Source: CAD feature listing. Evaluate the final solid. Frame: model axes, mm. A direction names the side the tool comes from. Give positions to 0.01 mm unless a question says otherwise; leave off trailing zeros. Write each loop counter-clockwise with the first axis right and the second up, starting at its lowest first coordinate (ties: lowest second). Pieces come first, ordered by that corner, then holes. Notation, with made-up numbers: (83.25, 41.5) -> (108.25, 41.5) arc R21 ccw to (108.25, 61.5) -> close; hole circle Ø8 at (-22.75, 50.25). An arc over 180 degrees is marked (long way). Answer as a JSON object with one key per item and string values. Group by question number.
Item 1: Pull-direction query (X, two-part tool) for faces 1 (the face through (25, 4, -7)), 2 (the face through (0, 7, 7)), 3 (the face through (14, 0, -5)); classes: pulls with the +X half, pulls with the -X half, needs draft (parallel to the pull), parting line crosses it, or undercut.
Item 2: Section query C-C on y = 7. Return the cut outline in (x, z).
Item 3: Access query for faces 4 (the face through (22, 12, -4)), 5 (the face through (40, 7, -6)), 6 (the face through (2.465, 5.388, 17.547)), 7 (the face through (25, 9.5, -8)), 8 (the face through (12.5, 7, -5)). Directions: +Z, -Z, +X, -X, +Y, -Y. A direction counts if a zero-diameter tool reaches every point of the face in a straight line with its end or side. Return the directions, or none.
Item 4: Section query A-A on x = 27. Return the cut outline in (y, z).
Item 5: Ray query, probe 1 along Y at (x, z) = (1.4, 3.65); probe 2 along X at (y, z) = (11, -3); probe 3 along Z at (x, y) = (31.5, 3). Return the intervals inside material, ascending. Write a range as from..to.
Item 6: First-contact query: pin 1 Ø1.6 at (x, z) = (29, -7.5) entering from -Y; pin 2 Ø5 at (y, z) = (7, 3.65) entering from +X; pin 3 Ø1.5 at (x, y) = (15.5, 4) entering from +Z; pin 4 Ø4 at (y, z) = (4, 12.5) entering from +X. Flat tips, straight axial feed; report the tip coordinate or a pass-through.
Item 7: Section query D-D on z = -5.5. Return the cut outline in (x, y), plus the area to 3 significant figures.
Item 8: Section query B-B on z = 3.65. Return the cut outline in (x, y).
from build123d import *

# Parameters (mm, degrees)
BOSS_EXTRUDE1_DEPTH  = 14
SKETCH2_W            = 25
SKETCH2_H            = 7
CUT_EXTRUDE3_DEPTH   = 3
SKETCH10_W           = 18
SKETCH10_H           = 5
CUT_EXTRUDE4_DEPTH   = 43.95346319
SKETCH20_W           = 24
SKETCH20_H           = 14
BOSS_EXTRUDE10_DEPTH = 5
SKETCH21_R           = 2.65
CUT_EXTRUDE13_DEPTH  = 5
SKETCH22_W           = 5
SKETCH22_H           = 4
CUT_EXTRUDE14_DEPTH  = 49.703182648
SKETCH23_R           = 2.65
BOSS_EXTRUDE11_DEPTH = 5


with BuildPart() as part:
    # Sketch1 → Boss-Extrude1 (new body)
    with BuildSketch(Plane(origin=(0, 0, 0), x_dir=(1, 0, 0), z_dir=(0, 1, 0))):
        Polygon((6.589095597, 0), (10, 0), (10, 4), (40, 4), (40, 9), (11.589095597, 9), (0, 9), (0, 0), align=None)
    extrude(amount=BOSS_EXTRUDE1_DEPTH)

    # Sketch2 → Cut-Extrude3 (cut)
    with BuildSketch(Plane.XY.offset(-4)):
        with Locations((25, 7)):
            Rectangle(SKETCH2_W, SKETCH2_H)
    extrude(amount=-CUT_EXTRUDE3_DEPTH, mode=Mode.SUBTRACT)

    # Sketch10 → Cut-Extrude4 (cut, through all)
    with BuildSketch(Plane.XY.offset(-7)):
        with Locations((25, 7)):
            Rectangle(SKETCH10_W, SKETCH10_H)
    extrude(amount=-CUT_EXTRUDE4_DEPTH, mode=Mode.SUBTRACT)

    # Sketch20 → Boss-Extrude10 (add)
    with BuildSketch(Plane.ZY):
        with Locations((12, 7)):
            Rectangle(SKETCH20_W, SKETCH20_H)
    extrude(amount=-BOSS_EXTRUDE10_DEPTH)

    # Sketch21 → Cut-Extrude13 (cut)
    with BuildSketch(Plane.ZY):
        with Locations((-4.35, 7)):
            Circle(SKETCH21_R)
        with Locations((3.65, 7)):
            Circle(SKETCH21_R)
        with Locations((11.65, 7)):
            Circle(SKETCH21_R)
        with Locations((19.65, 7)):
            Circle(SKETCH21_R)
    extrude(amount=-CUT_EXTRUDE13_DEPTH, mode=Mode.SUBTRACT)

    # Sketch22 → Cut-Extrude14 (cut, through all)
    with BuildSketch(Plane(origin=(0, 14, 0), x_dir=(1, 0, 0), z_dir=(0, 1, 0))):
        with Locations((7.5, 2)):
            Rectangle(SKETCH22_W, SKETCH22_H)
    extrude(amount=-CUT_EXTRUDE14_DEPTH, mode=Mode.SUBTRACT)

    # Sketch23 → Boss-Extrude11 (add)
    with BuildSketch(Plane.ZY):
        with Locations((-4.35, 7)):
            Circle(SKETCH23_R)
    extrude(amount=-BOSS_EXTRUDE11_DEPTH)


solid = part.part
Worked answers:
{
 "1": {"face 1": "undercut", "face 2": "pulls with the -X half", "face 3": "needs draft"},
 "2": {"outline": "(0, -9) -> (16, -9) -> (16, -7) -> (12.5, -7) -> (12.5, -4) -> (5, -4) -> (5, 1) -> (0, 1) -> close; (0, 6.3) -> (5, 6.3) -> (5, 9) -> (0, 9) -> close; (0, 14.3) -> (5, 14.3) -> (5, 17) -> (0, 17) -> close; (0, 22.3) -> (5, 22.3) -> (5, 24) -> (0, 24) -> close; (34, -9) -> (40, -9) -> (40, -4) -> (37.5, -4) -> (37.5, -7) -> (34, -7) -> close"},
 "3": {"face 4": "+Z, +X, +Y, -Y", "face 5": "+Z, -Z, +X, +Y, -Y", "face 6": "+X, -X", "face 7": "+Z, -Z", "face 8": "+Z"},
 "4": {"outline": "(0, -9) -> (4.5, -9) -> (4.5, -7) -> (3.5, -7) -> (3.5, -4) -> (0, -4) -> close; (9.5, -9) -> (14, -9) -> (14, -4) -> (10.5, -4) -> (10.5, -7) -> (9.5, -7) -> close"},
 "5": {"probe 1": "0..4.35, 9.65..14", "probe 2": "0..5", "probe 3": "-9..-4"},
 "6": {"pin 1": "y = 0", "pin 2": "through", "pin 3": "z = -4", "pin 4": "x = 5"},
 "7": {"outline": "(0, 0) -> (40, 0) -> (40, 14) -> (0, 14) -> close; hole (12.5, 3.5) -> (37.5, 3.5) -> (37.5, 10.5) -> (12.5, 10.5) -> close", "area": "385 mm^2"},
 "8": {"outline": "(0, 0) -> (5, 0) -> (5, 4.35) -> (0, 4.35) -> close; (0, 9.65) -> (5, 9.65) -> (5, 14) -> (0, 14) -> close"}
}
